from build123d import *

# Parameters (mm, degrees)
BOSS_EXTRUDE1_DEPTH                             = 2.925
CSK_FOR_M3_FLAT_HEAD_MACHINE_SCREW1_D           = 3.6
CSK_FOR_M3_FLAT_HEAD_MACHINE_SCREW1_CSINK_D     = 6.3
CSK_FOR_M3_FLAT_HEAD_MACHINE_SCREW1_CSINK_ANGLE = 90
FILLET1_R                                       = 2


with BuildPart() as part:
    # Sketch2 → Boss-Extrude1 (new body, symmetric)
    with BuildSketch(Plane(origin=(0, 0, 0), x_dir=(1, 0, 0), z_dir=(0, 1, 0))):
        with BuildLine():
            Line((-15, -4.875), (15, -4.875))
            Line((15, -4.875), (15, 4.875))
            Line((15, 4.875), (5.994789404, 4.875))
            ThreePointArc((5.994789404, 4.875), (0, -0.875), (-5.994789404, 4.875))
            Line((-5.994789404, 4.875), (-15, 4.875))
            Line((-15, 4.875), (-15, -4.875))
        make_face()
    extrude(amount=BOSS_EXTRUDE1_DEPTH, both=True)

    # CSK for M3 Flat Head Machine Screw1 (through all)
    with Locations(Plane.XY.offset(4.875)):
        with Locations((-10.497394702, 0), (10.497394702, 0)):
            CounterSinkHole(CSK_FOR_M3_FLAT_HEAD_MACHINE_SCREW1_D / 2, CSK_FOR_M3_FLAT_HEAD_MACHINE_SCREW1_CSINK_D / 2, counter_sink_angle=CSK_FOR_M3_FLAT_HEAD_MACHINE_SCREW1_CSINK_ANGLE)

    # Fillet1
    fillet1_edges = [part.edges().sort_by_distance(p)[0] for p in [
        (-15, 2.925, 0),
        (15, 2.925, 0),
        (15, -2.925, 0),
        (-15, -2.925, 0),
    ]]
    fillet(fillet1_edges, radius=FILLET1_R)


solid = part.part
Can you work these out from the model? Positions are in its coordinate system, mm. Give positions to 0.01 mm unless a question says otherwise; leave off trailing zeros. Order: outer loops, then holes, each group sorted by start corner. A loop starts at its lowest first (then second) coordinate and runs counter-clockwise, first axis right, second up. Notation, with made-up numbers: M -32.5,37.5 L -15.5,37.5 A36 cw -15.5,76.5 Z; hole C 21.25,54 d5. An arc over 180 degrees is marked long. Use a Markdown table: item, result. Add a question column.
Item 1: Suppose I cut it at D-D (z = -1.75). List the corners of the cut face in (x, y) for me (3 decimals), then the cut area to 3 significant figures.
Item 2: Suppose I cut it at B-B (z = -3.5). List the corners of the cut face in (x, y) for me (3 decimals), then the cut area to 3 significant figures.
Item 3: If I drill on L1, parallel to X at y = 0, z = 1.25; L2, parallel to X at y = 0, z = -1.5; L3, parallel to X at y = 0, z = -0.75, over which ranges is the centre line in solid material (lowest first)? Write a range as [from, to].
Item 4: We'd pull the mould along X, two halves only. Please class faces 1 (the flat face through (0, 2.925, 2)), 2 (the cylindrical face through (14.399, -2.355, -0.068)), 3 (the cylindrical face through (0.128, 0.041, 0.874)): +X half, -X half, draft (parallel to the pull), parting line (faces both ways), or undercut.
Item 5: Suppose I cut it at C-C (z = 2.5). List the corners of the cut face in (x, y) for me (3 decimals), then the cut area to 3 significant figures.
Item 6: Suppose I cut it at A-A (y = 0). List the corners of the cut face in (x, z) for me (3 decimals), then the cut area to 3 significant figures.
Item 7: Will this pin go through, and if not, where does the flat tip stop? pin 1 (3 mm diameter, centred on x = 10.5, y = 0, fed in from -Z).
Answer sheet:
| question | item | result |
|---|---|---|
| 1 | outline | M -15,-0.925 A2 ccw -13,-2.925 L -4.961,-2.925 L -4.961,2.925 L -13,2.925 A2 ccw -15,0.925 Z; M 4.961,-2.925 L 13,-2.925 A2 ccw 15,-0.925 L 15,0.925 A2 ccw 13,2.925 L 4.961,2.925 Z; hole C -10.497,0 d3.6; hole C 10.497,0 d3.6 |
| 1 | area | 93.7 mm² |
| 2 | outline | M -15,-0.925 A2 ccw -13,-2.925 L -5.776,-2.925 L -5.776,2.925 L -13,2.925 A2 ccw -15,0.925 Z; M 5.776,-2.925 L 13,-2.925 A2 ccw 15,-0.925 L 15,0.925 A2 ccw 13,2.925 L 5.776,2.925 Z; hole C -10.497,0 d3.6; hole C 10.497,0 d3.6 |
| 2 | area | 84.1 mm² |
| 3 | L1 | x = [-15, -12.3], [-8.7, 8.7], [12.3, 15] |
| 3 | L2 | x = [-15, -12.3], [-8.7, -4.78], [4.78, 8.7], [12.3, 15] |
| 3 | L3 | x = [-15, -12.3], [-8.7, -4.11], [4.11, 8.7], [12.3, 15] |
| 4 | face 1 | draft |
| 4 | face 2 | +X half |
| 4 | face 3 | undercut |
| 5 | outline | M -15,-0.925 A2 ccw -13,-2.925 L 13,-2.925 A2 ccw 15,-0.925 L 15,0.925 A2 ccw 13,2.925 L -13,2.925 A2 ccw -15,0.925 Z; hole C -10.497,0 d3.6; hole C 10.497,0 d3.6 |
| 5 | area | 152 mm² |
| 6 | outline | M -15,-4.875 L -12.297,-4.875 L -12.297,3.525 L -13.647,4.875 L -15,4.875 Z; M -8.697,-4.875 L -5.995,-4.875 A6 cw 5.995,-4.875 L 8.697,-4.875 L 8.697,3.525 L 7.347,4.875 L -7.347,4.875 L -8.697,3.525 Z; M 12.297,-4.875 L 15,-4.875 L 15,4.875 L 13.647,4.875 L 12.297,3.525 Z |
| 6 | area | 165 mm² |
| 7 | pin 1 | passes through |
